Autodesk Inventor part; units mm, degrees
ref_plane "YZ Plane" through (0, 0, 0) normal (1, 0, 0) x (0, 1, 0)
ref_plane "XZ Plane" through (0, 0, 0) normal (0, 1, 0) x (-1, 0, 0)
ref_plane "XY Plane" through (0, 0, 0) normal (0, 0, 1) x (1, 0, 0)
sketch "Sketch1" plane through (0, 0, 0) normal (0, 0, 1) x (1, 0, 0)
  line L0 (0, 0) -> (25, 0)
  line L1 (25, 0) -> (25, 40)
  line L2 (25, 40) -> (0, 40)
  line L3 (0, 40) -> (0, 0)
  dimension "d1" = 25
  dimension "d2" = 40
  dimension "d3" = 25
extrude "Extrusion1" add sketch "Sketch1" against normal blind 30
sketch "Sketch2" plane through (25, 0, 0) normal (1, 0, 0) x (0, 0, -1)
  line L0 (0, 0) -> (30, 0)
  circle A0 centre (15, 6.56) radius 2.46
extrude "Extrusion2" cut sketch "Sketch2" against normal blind 30
sketch "Sketch3" plane through (0, 0, 0) normal (-1, 0, 0) x (0, 0, 1)
  line L0 (0, 0) -> (-30, 0)
  line L1 (-25.05, 0) -> (-4.95, 0)
  line L2 (-4.95, 0) -> (-4.95, 33.12)
  line L3 (-4.95, 33.12) -> (-25.05, 33.12)
  line L4 (-25.05, 33.12) -> (-25.05, 0)
  dimension "d11" = 20.1
extrude "Extrusion3" cut sketch "Sketch3" against normal blind 20
sketch "Sketch4" plane through (0, 0, 0) normal (0, -1, 0) x (1, 0, 0)
  line L0 (20, -4.95) -> (20, -25.05)
  line L1 (20, -15) -> (25, -15)
  line L2 (25, 0) -> (25, -30)
  line L3 (20, -8.025) -> (25, -8.025)
  line L4 (25, -8.025) -> (25, -21.975)
  line L5 (25, -21.975) -> (20, -21.975)
  line L6 (20, -21.975) -> (20, -8.025)
  line L7 (20, -8.025) -> (25, -21.975) construction
  line L8 (25, -8.025) -> (20, -21.975) construction
  line L9 (25, -12.54) -> (25, -17.46)
  point P0 (0, 0)
  point P1 (22.5, -15)
  dimension "d14" = 13.95
extrude "Extrusion4" add sketch "Sketch4" along normal blind 15
sketch "Sketch5" plane through (20, 0, 0) normal (-1, 0, 0) x (0, 0, 1)
  circle A0 centre (-15, 6.56) radius 2.46
  circle A1 centre (-15, 6.56) radius 4.7025
  circle A2 centre (-15, 6.56) radius 2.46
  circle A3 centre (-15, 6.56) radius 2.46
  point P0 (0, 0)
  dimension "d17" = 9.405
extrude "Extrusion5" cut sketch "Sketch5" against normal blind 2.1
sketch "Sketch6" plane through (25, 0, 0) normal (1, 0, 0) x (0, 0, -1)
  circle A0 centre (15, 6.56) radius 4.7025
  line L0 (15, 6.56) -> (15, 23.56)
  circle A1 centre (15, 23.56) radius 2.46
  point P0 (0, 0)
  dimension "d20" = 17
  dimension "d21" = 4.92
extrude "Extrusion6" cut sketch "Sketch6" against normal blind 10 contours A1
sketch "Sketch7" plane through (20, 0, 0) normal (-1, 0, 0) x (0, 0, 1)
  circle A0 centre (-15, 23.56) radius 2.46
  circle A1 centre (-15, 23.56) radius 4.7025
  point P0 (0, 0)
  dimension "d24" = 9.405
extrude "Extrusion7" cut sketch "Sketch7" against normal blind 2.1
sketch "Sketch9" plane through (25, 0, 0) normal (1, 0, 0) x (0, 0, -1)
  circle A0 centre (15, 6.56) radius 2.46
  circle A1 centre (15, 6.56) radius 2.46
  circle A2 centre (15, 23.56) radius 2.46
  circle A3 centre (15, 23.56) radius 2.46
  line L0 (30, 40) -> (30, 0)
  line L1 (30, 0) -> (30, 40)
  line L2 (30, 40) -> (0, 40)
  line L3 (0, 40) -> (0, 0)
  line L4 (0, 0) -> (8.025, 0)
  line L5 (21.975, 0) -> (21.975, -15)
  line L6 (21.975, -15) -> (8.025, -15)
  line L7 (8.025, -15) -> (8.025, 0)
  line L8 (0, 0) -> (8.025, 0)
  line L9 (21.975, 0) -> (30, 0)
extrude "Extrusion8" add sketch "Sketch9" along normal blind 5
sketch "Sketch10" plane through (0, 40, 0) normal (0, 1, 0) x (1, 0, 0)
  line L0 (0, 30) -> (30, 30)
  line L1 (30, 0) -> (0, 0)
  line L2 (0, 30) -> (30, 30)
  line L3 (30, 30) -> (30, 0)
  line L4 (30, 0) -> (0, 0)
  line L5 (0, 0) -> (0, 30)
extrude "Extrusion9" add sketch "Sketch10" along normal blind 30
sketch "Sketch12" plane through (30, 0, 0) normal (1, 0, 0) x (0, 0, -1)
  circle A0 centre (15, 6.56) radius 2.46
  line L0 (15, 6.56) -> (15, 15.06)
  circle A1 centre (15, 15.06) radius 2.525
  point P0 (0, 0)
  dimension "d31" = 8.5
  dimension "d33" = 5.05
extrude "Extrusion10" cut sketch "Sketch12" against normal blind 30 contours A1
sketch "Sketch14" plane through (0, 0, 0) normal (0, 0, 1) x (1, 0, 0)
  line L0 (30, 70) -> (0, 70)
  line L1 (0, 70) -> (0, 85)
  line L2 (30, 0) -> (30, 70)
  line L3 (30, 109) -> (30, 70)
  line L4 (30, 105) -> (30, 100)
  line L5 (-12, 124) -> (15, 124)
  line L6 (-8, 122) -> (-12, 124)
  line L7 (-8, 122) -> (-4, 112)
  line L8 (-8, 102) -> (-12, 100)
  line L9 (-8, 102) -> (-4, 112)
  line L10 (30, 109) -> (15, 124)
  line L11 (0, 85) -> (0, 100)
  line L12 (0, 100) -> (-12, 100)
  point P0 (0, 0)
  dimension "d69" = 12
extrude "Extrusion12" add sketch "Sketch14" against normal blind 30
sketch "Sketch15" plane through (0, 0, -25.05) normal (-1, 0, 0) x (0, 0, 1)
  line L0 (0, 33.12) -> (20.1, 33.12)
  line L1 (20.1, 33.12) -> (20.1, 0)
  line L2 (0, 33.12) -> (20.1, 33.12)
  line L3 (20.1, 33.12) -> (20.1, 31.1)
  line L4 (20.1, 31.1) -> (0, 31.1)
  line L5 (0, 31.1) -> (0, 33.12)
  point P0 (25.05, 0)
  dimension "d57" = 2.02
extrude "Extrusion13" add sketch "Sketch15" against normal blind 20
properties part number "20mm_x_30mm"
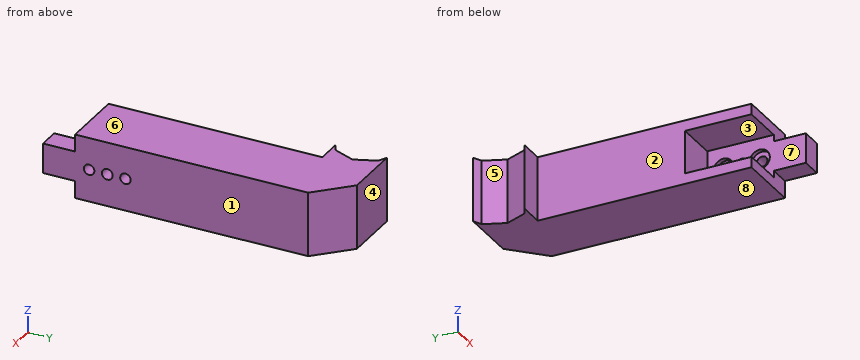
CAD build for the part. Positions are in the model's coordinates, mm. Face numbers are marked on the shaded views. A direction names the side the tool comes from. Round coordinates to 2 decimals unless told otherwise and drop trailing zeros. Order: outer loops, then holes, each group sorted by start corner. A loop starts at its lowest first (then second) coordinate and runs counter-clockwise, first axis right, second up. Notation, with made-up numbers: (79, -38.5) - (106, -38.5) arc R19 ccw to (106, -30.5) - close; hole circle Ø7 at (87.25, 59). An arc over 180 degrees is marked (long way). Use CSV: the item, a comma, the result in double quotes. Start each with the question number.
1) Saw through at A-A (y = 15.06). List the corners of the cut face in (x, z) (3 decimals), and give its area (4 significant figures).
2) Saw through at C-C (y = 58.5). List the corners of the cut face in (x, z), and give its area (3 significant figures).
3) Saw through at B-B (z = -15). Count the separate pieces of the cut face and the enclosed holes in it, and give its area (3 significant figures).
4) Two-plate mould, pull along Z, no slides. Class the marked faces 6, 7 and 8: pulls with the +Z half, pulls with the -Z half, needs draft (parallel to the pull), parting line crosses it, or undercut.
5) Tool access for the marked faces 1, 2, 3, 4 and 5: list every direction of +Z, -Z, +X, -X, +Y, -Y with a clear straight run to the whole face (end or side of a thin tool).
6) Pin check, flat tips, straight feed: pin 1 Ø16 at (y, z) = (7.5, -14) entering from -X; pin 2 Ø4.5 at (y, z) = (6.56, -15) entering from -X; pin 3 Ø4 at (x, z) = (21, -25) entering from -Y; pin 4 Ø4 at (y, z) = (47, -12) entering from -X. Stop position of each tip, or through.
7) Wall check: L1, parallel to Z at x = 24.75, y = 6.56; L2, parallel to Y at x = 24.75, z = -15 (3 decimals); L3, parallel to Y at x = 23.5, z = -15 (3 decimals). Give the ranges that are in metal, low to high. Write a range as [from, to].
Values follow:
1,outline,"(0, -30) - (30, -30) - (30, -17.525) - (20, -17.525) - (20, -25.05) - (0, -25.05) - close; (0, -4.95) - (20, -4.95) - (20, -12.475) - (30, -12.475) - (30, 0) - (0, 0) - close"
1,area,"447.5 mm2"
2,outline,"(0, -30) - (30, -30) - (30, 0) - (0, 0) - close"
2,area,"900 mm2"
3,separate pieces,"4"
3,enclosed holes,"0"
3,area,"3,130 mm2"
4,face 6,"pulls with the +Z half"
4,face 7,"undercut"
4,face 8,"pulls with the -Z half"
5,face 1,"+Z, -Z, +X, +Y, -Y"
5,face 2,"+Z, -Z, -X, -Y"
5,face 3,"-X, -Y"
5,face 4,"+Z, -Z, +X, -X, +Y"
5,face 5,"+Z, -Z, -X"
6,pin 1,"stops at x = 20"
6,pin 2,"passes through"
6,pin 3,"stops at y = 0"
6,pin 4,"stops at x = 0"
7,L1,"z = [-30, -17.46], [-12.54, 0]"
7,L2,"y = [-15, 4.1], [9.02, 12.535], [17.585, 21.1], [26.02, 114.25]"
7,L3,"y = [-15, 4.1], [9.02, 12.535], [17.585, 21.1], [26.02, 115.5]"
